from build123d import *

# Parameters (mm, degrees)
F1_DEPTH = 1.8
F2_R     = 0.5
F3_SIZE  = 0.5


with BuildPart() as f1:
    # F0 (on Top) → F1 (new body)
    with BuildSketch(Plane.XY):
        Polygon((-5.25, -15), (5.25, -15), (5.25, 15), (2, 15), (2, 23), (0, 23), (-2, 23), (-2, 15), (-5.25, 15), align=None)
    extrude(amount=F1_DEPTH)

    # F2
    f2_edges = [f1.edges().sort_by_distance(p)[0] for p in [
        (2, 23, 0.9),
        (-2, 23, 0.9),
        (5.25, 15, 0.9),
        (-5.25, 15, 0.9),
    ]]
    fillet(f2_edges, radius=F2_R)

    # F3
    f3_edges = [f1.edges().sort_by_distance(p)[0] for p in [
        (0, -15, 0),
        (0, -15, 1.8),
        (5.25, -15, 0.9),
        (-5.25, -15, 0.9),
    ]]
    chamfer(f3_edges, length=F3_SIZE)


solid = f1.part
Verification items for the finished model (mm, model axes). A direction names the side the tool comes from. Coordinates: 2 decimals unless noted, no trailing zeros. Order: outer loops, then holes, each group sorted by start corner. A loop starts at its lowest first (then second) coordinate and runs counter-clockwise, first axis right, second up. Notation, with made-up numbers: M -2,34.25 L 48,34.25 A26 cw 48,65.25 Z; hole C -13,38.5 d6. An arc over 180 degrees is marked long. One line per item, written item: value. Start each with the question number.
Item 1: Sectioned sample at A-A (x = 3.5). Enter the section's corners in (y, z).
Item 2: Access from +Z, -Z, +X, -X, +Y, -Y to the whole of each face (thin tool, end or side, straight path). Record for faces 1 (the flat face through (0, 23, 1)), 2 (the flat face through (-3, 15, 1)), 3 (the flat face through (3, 15, 1)).
Item 3: Sectioned sample at B-B (y = 15.5). Enter the section's corners in (x, z).
Item 4: Scan lines: probe 1 along Y at (x, z) = (2.25, 0.6); probe 2 along X at (y, z) = (17.5, 1.2); probe 3 along Y at (x, z) = (0, 1.65). Record each from-to range of solid material in increasing order.
Item 5: Gauge pin test, flat ends, axial feed: pin 1 (0.9 mm diameter, centred on x = -4, z = 1, fed in from +Y); pin 2 (0.5 mm diameter, centred on y = 19, z = 0.5, fed in from -X). Record the tip position at first contact, or that the pin passes through.
Conclusion:
1. outline: M -15,0.5 L -14.5,0 L 15,0 L 15,1.8 L -14.5,1.8 L -15,1.3 Z
2. face 1: +Z, -Z, +X, -X, +Y
2. face 2: +Z, -Z, -X, +Y
2. face 3: +Z, -Z, +X, +Y
3. outline: M -2,0 L 2,0 L 2,1.8 L -2,1.8 Z
4. probe 1: y = -15 to 15
4. probe 2: x = -2 to 2
4. probe 3: y = -14.65 to 23
5. pin 1: stops at y = 15
5. pin 2: stops at x = -2
